```python
from build123d import *

# Parameters (mm, degrees)
BOSS_EXTRUDE1_DEPTH = 84.0232
SKETCH2_R           = 5.969
CUT_EXTRUDE1_DEPTH  = 0.7366
LPATTERN1_COUNT     = 2
LPATTERN1_PITCH     = 80.1116


with BuildPart() as part:
    # Sketch1 → Boss-Extrude1 (new body)
    with BuildSketch(Plane.XY.offset(31.75)):
        Polygon((7.332348419, 0), (3.666174209, 6.35), (-3.666174209, 6.35), (-7.332348419, 0), (-3.666174209, -6.35), (3.666174209, -6.35), align=None)
    extrude(amount=-BOSS_EXTRUDE1_DEPTH)

    # Sketch2 → Cut-Extrude1 (cut)
    with BuildSketch(Plane.XY.offset(30.1625)):
        Polygon((-3.666174209, -6.35), (3.666174209, -6.35), (7.332348419, 0), (3.666174209, 6.35), (-3.666174209, 6.35), (-7.332348419, 0), align=None)
        Circle(SKETCH2_R, mode=Mode.SUBTRACT)
    cut_extrude1 = extrude(amount=-CUT_EXTRUDE1_DEPTH, mode=Mode.SUBTRACT)

    # LPattern1: Cut-Extrude1 ×2
    with Locations(*[(0, 0, -i * LPATTERN1_PITCH) for i in range(1, LPATTERN1_COUNT)]):
        add(cut_extrude1, mode=Mode.SUBTRACT)


solid = part.part
```
Check sheet for the modelled part. Datum: model origin and axes. Units: mm. A direction names the side the tool comes from. Give positions to 0.01 mm unless a question says otherwise; leave off trailing zeros. Loops run counter-clockwise (first coordinate to the right, second up) from the corner with the lowest first, then second, coordinate; pieces in that order, holes last. Notation, with made-up numbers: M 5,42.5 L 59,42.5 A6 ccw 59,53.5 Z; hole C -7,58.25 d11. An arc over 180 degrees is marked long. Answer as CSV lines item,"result".
Item 1: Sectioned sample at A-A, the plane y = -4. Enter the section's corners in (x, z).
Reply:
outline,"M -5.02,-52.27 L 5.02,-52.27 L 5.02,-50.69 L 4.43,-50.69 L 4.43,-49.95 L 5.02,-49.95 L 5.02,29.43 L 4.43,29.43 L 4.43,30.16 L 5.02,30.16 L 5.02,31.75 L -5.02,31.75 L -5.02,30.16 L -4.43,30.16 L -4.43,29.43 L -5.02,29.43 L -5.02,-49.95 L -4.43,-49.95 L -4.43,-50.69 L -5.02,-50.69 Z"
Item 2: Scan lines: L1, parallel to Y at x = -3.75, z = -32.5; L2, parallel to X at y = -2.25, z = -0.5; L3, parallel to X at y = 4.5, z = -12. Record each from-to range of solid material in increasing order.
Reply:
L1,"-6.2 to 6.2"
L2,"-6.03 to 6.03"
L3,"-4.73 to 4.73"
Item 3: Sectioned sample at B-B, the plane z = -16.5. Enter the section's corners in (x, y).
Reply:
outline,"M -7.33,0 L -3.67,-6.35 L 3.67,-6.35 L 7.33,0 L 3.67,6.35 L -3.67,6.35 Z"
Item 4: Sectioned sample at C-C, the plane y = 3.5. Enter the section's corners in (x, z).
Reply:
outline,"M -5.31,-52.27 L 5.31,-52.27 L 5.31,-50.69 L 4.84,-50.69 L 4.84,-49.95 L 5.31,-49.95 L 5.31,29.43 L 4.84,29.43 L 4.84,30.16 L 5.31,30.16 L 5.31,31.75 L -5.31,31.75 L -5.31,30.16 L -4.84,30.16 L -4.84,29.43 L -5.31,29.43 L -5.31,-49.95 L -4.84,-49.95 L -4.84,-50.69 L -5.31,-50.69 Z"
Item 5: Draft check along Z on faces 3 (the face through (-5.525, -3.131, 30.967)), 4 (the face through (5.4, 2.9, -49.949)), 5 (the face through (0, 0, -52.273)), 6 (the face through (0, 0, 31.75)). Enter one of: pulls with the +Z half, pulls with the -Z half, needs draft (parallel to the pull), parting line crosses it, or undercut.
Reply:
face 3,"needs draft"
face 4,"undercut"
face 5,"pulls with the -Z half"
face 6,"pulls with the +Z half"
Item 6: Set-up check for faces 1 (the face through (5.4, 2.9, 30.162)), 2 (the face through (5.525, 3.131, -9.706)): record each of +Z, -Z, +X, -X, +Y, -Y from which the full face is reachable in a straight line by a thin tool's end or side.
Reply:
face 1,"none"
face 2,"+Z, -Z, +X, +Y"
